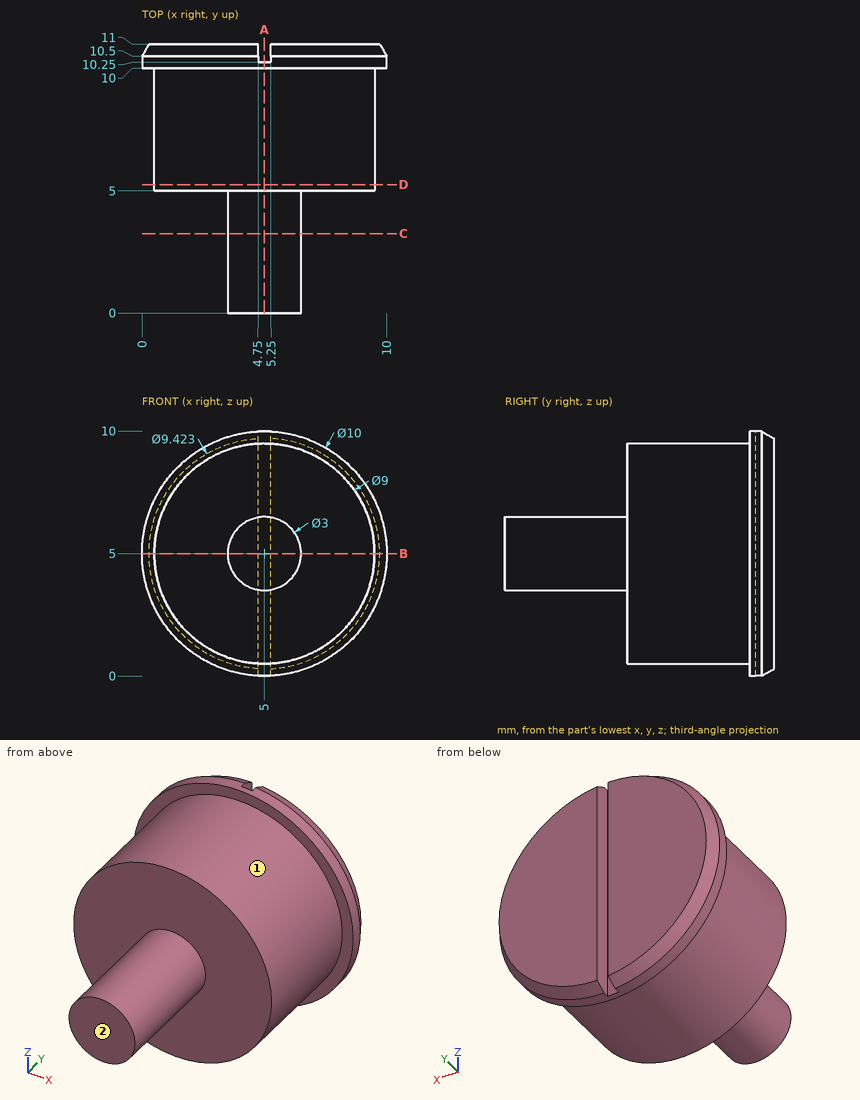
The drawing under review shows one solid part. Ordinate dimensions are in mm from its lowest x, y, z. A direction names the side the tool comes from. Coordinates: 2 decimals unless noted, no trailing zeros. Write each loop counter-clockwise with the first axis right and the second up, starting at its lowest first coordinate (ties: lowest second). Pieces come first, ordered by that corner, then holes. Notation, with made-up numbers: (88, 5) - (125, 5) arc R13 ccw to (125, 11) - close; hole circle Ø3 at (78.5, 55.25). An arc over 180 degrees is marked (long way). Use one line per item in the form item = value.
Q1. Consider section D-D (y = 5.25). Write out the cut boundary in (x, z), plus the area to 3 significant figures.
Taken from the geometry:
outline = circle Ø9 at (5, 5)
area = 63.6 mm^2
Q2. Machinability: for the marked faces 1 and 2, which of the approach directions +Z, -Z, +X, -X, +Y, -Y give a long, thin tool a straight path to every point of the face, cutting with its end or side? Answer none if there is none.
Taken from the geometry:
face_1 = -Y
face_2 = +Z, -Z, +X, -X, -Y
Q3. Consider section B-B (z = 5). Write out the cut boundary in (x, y), plus the area to 3 significant figures.
Taken from the geometry:
outline = (0, 10) - (0.5, 10) - (0.5, 5) - (3.5, 5) - (3.5, 0) - (6.5, 0) - (6.5, 5) - (9.5, 5) - (9.5, 10) - (10, 10) - (10, 10.5) - (9.71, 11) - (5.25, 11) - (5.25, 10.25) - (4.75, 10.25) - (4.75, 11) - (0.29, 11) - (0, 10.5) - close
area = 69.5 mm^2
Q4. For probe 1 along Y at (x, z) = (3, 8); probe 2 along Z at (x, y) = (5, 1.5); probe 3 along Y at (x, z) = (1, 2.75), list the stretches that pass through material, from the lowest coordinate up.
Taken from the geometry:
probe_1 = 5 to 11
probe_2 = 3.5 to 6.5
probe_3 = 10 to 11
Q5. Consider section C-C (y = 3.25). Write out the cut boundary in (x, z).
Taken from the geometry:
outline = circle Ø3 at (5, 5)
Q6. Insertion check: pin 1 Ø5 at (x, y) = (3, 5) entering from -Z; pin 2 Ø5 at (y, z) = (6.5, 2) entering from -X; pin 3 Ø4 at (x, z) = (3.5, 1) entering from -Y. Each pin has a flat end and moves straight along its axis. Give the tip position at first contact, or say it passes through.
Taken from the geometry:
pin_1 = 0.5
pin_2 = 0.53
pin_3 = 5
Q7. Consider section A-A (x = 5). Write out the cut boundary in (y, z), plus the area to 3 significant figures.
Taken from the geometry:
outline = (0, 3.5) - (5, 3.5) - (5, 0.5) - (10, 0.5) - (10, 0) - (10.25, 0) - (10.25, 10) - (10, 10) - (10, 9.5) - (5, 9.5) - (5, 6.5) - (0, 6.5) - close
area = 62.5 mm^2
